from build123d import *

# Parameters (mm, degrees)
ESQUISSE1_W        = 20
ESQUISSE1_H        = 5
BOSS_EXTRU_1_DEPTH = 5


with BuildPart() as part:
    # Esquisse1 → Boss.-Extru.1 (new body)
    with BuildSketch(Plane.XY):
        Polygon((-100, 150), (100, 150), (100, 90), (105, 90), (105, 150), (113, 150), (113, 0), (-113, 0), (-113, 150), (-105, 150), (-105, 90), (-100, 90), align=None)
        with Locations((90, 7.5)):
            Rectangle(ESQUISSE1_W, ESQUISSE1_H, mode=Mode.SUBTRACT)
        with Locations((90, 77.5)):
            Rectangle(ESQUISSE1_W, ESQUISSE1_H, mode=Mode.SUBTRACT)
        Polygon((-15, 5), (15, 5), (15, 10), (0, 10), (-15, 10), align=None, mode=Mode.SUBTRACT)
        Polygon((-15, 80), (0, 80), (15, 80), (15, 75), (-15, 75), align=None, mode=Mode.SUBTRACT)
        with Locations((-90, 7.5)):
            Rectangle(ESQUISSE1_W, ESQUISSE1_H, mode=Mode.SUBTRACT)
        with Locations((-90, 77.5)):
            Rectangle(ESQUISSE1_W, ESQUISSE1_H, mode=Mode.SUBTRACT)
    extrude(amount=BOSS_EXTRU_1_DEPTH)


solid = part.part
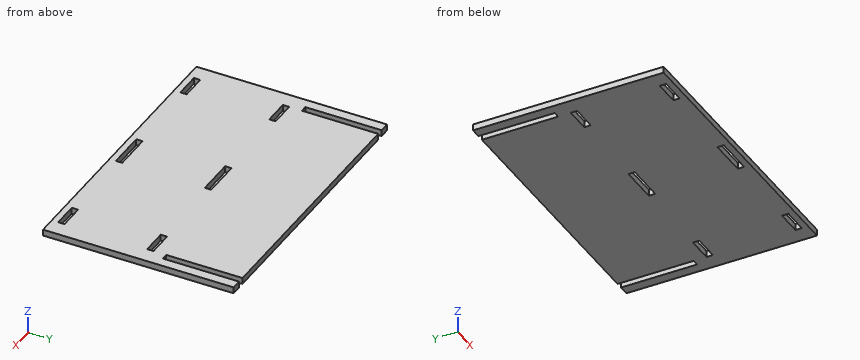
Read the model definition and answer for the solid it produces. Units are mm, in the model's axes. Coordinates: 2 decimals unless noted, no trailing zeros. Order: outer loops, then holes, each group sorted by start corner. A loop starts at its lowest first (then second) coordinate and runs counter-clockwise, first axis right, second up. Notation, with made-up numbers: (-23.5, 7.25) - (-17.5, 7.25) arc R20 cw to (-17.5, 45.25) - close; hole circle Ø2 at (4.25, -35). An arc over 180 degrees is marked (long way). Use one line per item in the form item = value.
(1) Given pin 1 Ø1.5 at (x, z) = (-90, 1.5) entering from -Y, flat-ended and moving along its own axis, determine where the tip first touches the part or whether it passes through.
Computed values:
pin_1 = 0
(2) Section B-B, the plane x = 9 is taken. Give the vertices of the cut face in (y, z).
Computed values:
outline = (0, 0) - (5, 0) - (5, 5) - (0, 5) - close; (10, 0) - (75, 0) - (75, 5) - (10, 5) - close; (80, 0) - (150, 0) - (150, 5) - (80, 5) - close
(3) Section A-A, the plane y = 136.5 is taken. Give the vertices of the cut face in (x, z).
Computed values:
outline = (-113, 0) - (-105, 0) - (-105, 5) - (-113, 5) - close; (-100, 0) - (100, 0) - (100, 5) - (-100, 5) - close; (105, 0) - (113, 0) - (113, 5) - (105, 5) - close
(4) Straight lines are drawn through the part: L1, parallel to Y at x = 4.5, z = 3.7; L2, parallel to X at y = 6, z = 2.6; L3, parallel to X at y = 103, z = 1.75. For each, find the intervals that lie inside material, in ascending order.
Computed values:
L1 = 0 to 5, 10 to 75, 80 to 150
L2 = -113 to -100, -80 to -15, 15 to 80, 100 to 113
L3 = -113 to -105, -100 to 100, 105 to 113
(5) Section C-C, the plane z = 3.85 is taken. Give the number of separate pieces and of enclosed holes in the cut face, then the cut area to 3 significant figures.
Computed values:
separate_pieces = 1
enclosed_holes = 6
area = 32,600 mm²
